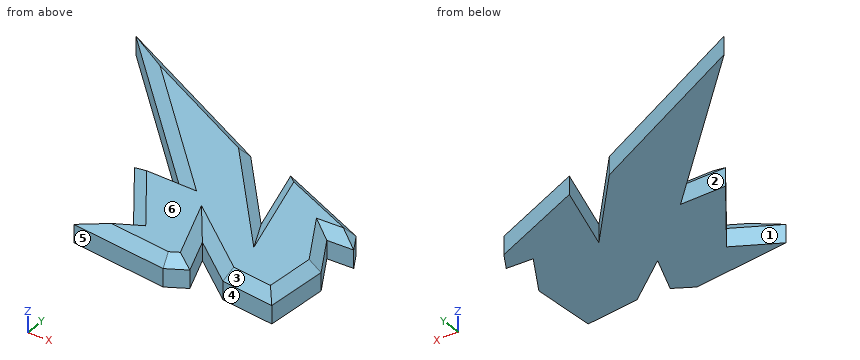
from build123d import *

# Parameters (mm, degrees)
F1_DEPTH = 12.7
F2_SIZE  = 4.572


# Not quite as in the source:
# - a feature names something its author has since deleted; it is built from what else it names


with BuildPart() as f1:
    # F0 (on Top) → F1 (new body)
    with BuildSketch(Plane.XY):
        Polygon((-47.4197901785, 9.0821487829), (-54.1167072952, 27.1118637174), (-33.1560820341, 9.7886463627), (-9.0490672737, 6.4328033477), (-6.5208841115, 34.9811986089), (-16.9482622296, 54.0015585721), (-5.0941226073, 54.2380437255), (-9.5673697069, 62.3648315668), (-52.2826313972, 82.1464285254), (-43.0134832859, 49.2380969226), (-71.8594374871, 84.6780897401), (-152.3833320228, 127.5459273348), (-82.3831111193, 53.5424649715), (-102.9803976417, 54.3163046241), (-80.3189948201, 20.4314347357), (-100.0030711293, 10.3000625968), (-56.1285279691, 4.3535600416), align=None)
    extrude(amount=F1_DEPTH)

    # F2
    f2_edges = [f1.edges().sort_by_distance(p)[0] for p in [
        (-30.925001, 72.25563, 12.7),
        (-47.648057, 65.692263, 12.7),
        (-57.43646, 66.958093, 12.7),
        (-112.121385, 106.112009, 12.7),
        (-117.383222, 90.544196, 12.7),
        (-92.681754, 53.929385, 12.7),
        (-91.649696, 37.37387, 12.7),
        (-90.161033, 15.365749, 12.7),
        (-78.0658, 7.326811, 12.7),
        (-51.774159, 6.717854, 12.7),
        (-50.768249, 18.097006, 12.7),
        (-43.636395, 18.450255, 12.7),
        (-21.102575, 8.110725, 12.7),
        (-7.784976, 20.707001, 12.7),
        (-11.734573, 44.491379, 12.7),
        (-11.021192, 54.119801, 12.7),
        (-7.330746, 58.301438, 12.7),
    ]]
    chamfer(f2_edges, length=F2_SIZE)


solid = f1.part
Design review of the part built by this model. Coordinates are the model's own, in mm. Face numbers are marked on the shaded views. A direction names the side the tool comes from. Coordinates: 2 decimals unless noted, no trailing zeros. Order: outer loops, then holes, each group sorted by start corner. A loop starts at its lowest first (then second) coordinate and runs counter-clockwise, first axis right, second up.
Item 1: Take a section at B-B, the plane z = 2. Write out the cut boundary in (x, y).
Item 2: For line 1 (X direction, y = 81, z = 4.75); line 2 (X direction, y = 22, z = 1.5); line 3 (Y direction, x = -128, z = 3), list the stretches that pass through material, from the lowest coordinate up.
Item 3: For pin 1 Ø1 at (y, z) = (26.5, 5) entering from +X; pin 2 Ø4 at (x, z) = (-131.5, 9) entering from -Y; pin 3 Ø1.5 at (x, z) = (-82.5, 11) entering from -Y, all flat-tipped, find the tip position at first contact; note any pin that passes through.
Item 4: The part is to be moulded in two halves that separate along X. For the marked faces 4, 5 and 6, say which applies: pulls with the +X half, pulls with the -X half, needs draft (parallel to the pull), parting line crosses it, or undercut.
Item 5: Take a section at A-A, the plane x = -91. Write out the cut boundary in (y, z), then the cut area to 3 significant figures.
Item 6: For the marked faces 1, 2 and 3, list the 3-axis set-ups (+Z, -Z, +X, -X, +Y, -Y) from which the entire face can be reached by the end or side of a thin tool; tool diameter is ignored.
Item 7: Take a section at C-C, the plane y = 117. Write out the cut boundary in (x, z).
Item 8: Take a section at D-D, the plane x = -139. Write out the cut boundary in (y, z), then the cut area to 3 significant figures.
The answers:
1. outline: (-152.38, 127.55) - (-82.38, 53.54) - (-102.98, 54.32) - (-80.32, 20.43) - (-100, 10.3) - (-56.13, 4.35) - (-47.42, 9.08) - (-54.12, 27.11) - (-33.16, 9.79) - (-9.05, 6.43) - (-6.52, 34.98) - (-16.95, 54) - (-5.09, 54.24) - (-9.57, 62.36) - (-52.28, 82.15) - (-43.01, 49.24) - (-71.86, 84.68) - close
2. line 1: x = -108.36 to -68.87, -51.96 to -49.81
2. line 2: x = -81.37 to -52.22, -47.93 to -7.67
2. line 3: y = 101.77 to 114.57
3. pin 1: stops at x = -7.23
3. pin 2: stops at y = 103.57
3. pin 3: stops at y = 10.06
4. face 4: undercut
4. face 5: pulls with the -X half
4. face 6: needs draft
5. outline: (9.08, 0) - (14.93, 0) - (14.93, 8.13) - (11.85, 10.87) - (9.08, 8.13) - close; (36.4, 0) - (53.87, 0) - (53.87, 8.13) - (49.29, 12.7) - (44.63, 12.7) - (36.4, 8.13) - close; (62.65, 0) - (94.87, 0) - (94.87, 8.13) - (89.69, 12.7) - (69.31, 12.7) - (62.65, 8.13) - close
5. area: 630 mm2
6. face 1: +Z, -Z, -X
6. face 2: +Z, -Z
6. face 3: +Z, -Y
7. outline: (-142.41, 0) - (-132.57, 0) - (-132.57, 8.13) - (-138.55, 10.93) - (-142.41, 8.13) - close
8. outline: (113.4, 0) - (120.42, 0) - (120.42, 8.13) - (117.35, 10.84) - (113.4, 8.13) - close
8. area: 66.6 mm2
